Check sheet for the modelled part. Datum: model origin and axes. Units: mm. A direction names the side the tool comes from. Coordinates: 2 decimals unless noted, no trailing zeros. Loops run counter-clockwise (first coordinate to the right, second up) from the corner with the lowest first, then second, coordinate; pieces in that order, holes last. Notation, with made-up numbers: M 20.25,81.25 L 29.25,81.25 A27 cw 29.25,111.25 Z; hole C 70,39 d2. An arc over 180 degrees is marked long. Answer in a Markdown table with one row per item. Add a question column.
Autodesk Inventor part; units mm, degrees
ref_plane "YZ Plane" through (0, 0, 0) normal (1, 0, 0) x (0, 1, 0)
ref_plane "XZ Plane" through (0, 0, 0) normal (0, 1, 0) x (-1, 0, 0)
ref_plane "XY Plane" through (0, 0, 0) normal (0, 0, 1) x (1, 0, 0)
sketch "スケッチ1" plane through (0, 0, 0) normal (0, 0, 1) x (1, 0, 0)
  circle A0 centre (0, 0) radius 1.5
  dimension "d0" = 3
extrude "押し出し1" add sketch "スケッチ1" along normal blind 6
sketch "スケッチ2" plane through (0, 0, 6) normal (0, 0, 1) x (1, 0, 0)
  circle A0 centre (0, 0) radius 1.5
  circle A1 centre (0, 0) radius 3
  dimension "d3" = 6
extrude "押し出し2" add sketch "スケッチ2" along normal blind 1.75 contours A0 | A1
thread "ねじ1"
chamfer "面取り1" distance 1.5 angle 45 1 edges at (-3, 0, 6)
sketch "スケッチ4" plane through (0, 0, 0) normal (0, 0, -1) x (-1, 0, 0)
  circle A0 centre (0, 0) radius 1.5
extrude "押し出し4" cut sketch "スケッチ4" against normal blind 1.75
properties part number "SB　6mm皿ネジ" material "Steel, Mild"
Q1. Access from +Z, -Z, +X, -X, +Y, -Y to the whole of each face (thin tool, end or side, straight path). Record for faces 1 (the face through (-1.5, -0.07, 3.85)), 2 (the face through (0, 0, 7.75)).
Q2. Go/stop test with a flat-tipped pin: pin 1 (3 mm diameter, centred on x = -0.5, z = 4, fed in from -Y). Record where the tip stops, or that it passes through.
Q3. Cross-section at C-C (z = 2.6). Record the cut outline in (x, y).
Q4. Thickness scan on L1, parallel to Y at x = 0.4, z = 7.2; L2, parallel to Y at x = -1.1, z = 3.25; L3, parallel to Z at x = -0.1, y = 2.05. Record the ranges inside material, lowest first.
Answer key:
| question | item | result |
|---|---|---|
| 1 | face 1 | -Z |
| 1 | face 2 | +Z, +X, -X, +Y, -Y |
| 2 | pin 1 | y = -1.5 |
| 3 | outline | C 0,0 d3 |
| 4 | L1 | -2.67 to 2.67 |
| 4 | L2 | -1.02 to 1.02 |
| 4 | L3 | 6.55 to 7.75 |
